CAD build for the part. Positions are in the model's coordinates, mm. Coordinates: 2 decimals unless noted, no trailing zeros. Order: outer loops, then holes, each group sorted by start corner. A loop starts at its lowest first (then second) coordinate and runs counter-clockwise, first axis right, second up. Notation, with made-up numbers: M -9.5,40.25 L -3.5,40.25 A11 cw -3.5,53.25 Z; hole C -14,36.25 d10. An arc over 180 degrees is marked long. Write item = value, one per line. Start each with the question number.
```python
from build123d import *

# Parameters (mm, degrees)
SKETCH1_R           = 317.5
SKETCH1_R_2         = 47.5
BOSS_EXTRUDE1_DEPTH = 5
SKETCH2_R           = 6
CUT_EXTRUDE1_DEPTH  = 5
CIRPATTERN1_COUNT   = 12
SKETCH6_R           = 3
CUT_EXTRUDE2_DEPTH  = 10
CIRPATTERN2_COUNT   = 3


with BuildPart() as part:
    # Sketch1 → Boss-Extrude1 (new body)
    with BuildSketch(Plane(origin=(0, 0, 0), x_dir=(0, 0, -1), z_dir=(1, 0, 0))):
        Circle(SKETCH1_R)
        Circle(SKETCH1_R_2, mode=Mode.SUBTRACT)
    extrude(amount=BOSS_EXTRUDE1_DEPTH)

    # Sketch2 → Cut-Extrude1 (cut)
    with BuildSketch(Plane(origin=(5, 0, 0), x_dir=(0, 0, -1), z_dir=(1, 0, 0))):
        with Locations((300, 0)):
            Circle(SKETCH2_R)
    cut_extrude1 = extrude(amount=-CUT_EXTRUDE1_DEPTH, mode=Mode.SUBTRACT)

    # CirPattern1: Cut-Extrude1 ×12 about axis
    cirpattern1_axis = Axis((0, 0, 0), (1, 0, 0))
    for i in range(1, CIRPATTERN1_COUNT):
        add(cut_extrude1.rotate(cirpattern1_axis, i * 360 / CIRPATTERN1_COUNT), mode=Mode.SUBTRACT)

    # Sketch6 → Cut-Extrude2 (cut)
    with BuildSketch(Plane(origin=(5, 0, 0), x_dir=(0, 0, -1), z_dir=(1, 0, 0))):
        with Locations((0, 55)):
            Circle(SKETCH6_R)
    cut_extrude2 = extrude(amount=-CUT_EXTRUDE2_DEPTH, mode=Mode.SUBTRACT)

    # CirPattern2: Cut-Extrude2 ×3 about axis
    cirpattern2_axis = Axis((0, 0, 0), (1, 0, 0))
    for i in range(1, CIRPATTERN2_COUNT):
        add(cut_extrude2.rotate(cirpattern2_axis, i * 360 / CIRPATTERN2_COUNT), mode=Mode.SUBTRACT)


solid = part.part
```
1. Probe L1, parallel to Y at x = 3, z = 5.5; L2, parallel to Y at x = 2.9, z = 150; L3, parallel to Y at x = 2.1, z = 43. List the from-to ranges inside material, lowest first.
2. Flat gauge pins, fed straight in: pin 1 (7 mm diameter, centred on y = -27.5, z = -47.63, fed in from -X); pin 2 (1.5 mm diameter, centred on x = 4, y = 171.5, fed in from -Z); pin 3 (1 mm diameter, centred on x = 1, z = 212.5, fed in from +Y); pin 4 (1 mm diameter, centred on x = 1.5, y = -27, fed in from +Z). Where does each tip first touch, or does it go through?
3. Slice it at A-A (x = 0.9). Give the number of separate pieces and of enclosed holes in the cut face, plus the area to 3 significant figures.
4. Slice it at C-C (y = -188.5). Write the cut outline in (x, z), plus the area to 3 significant figures.
5. Slice it at B-B (z = -242). Write the cut outline in (x, y).
Calculated:
q1.L1 = -317.45 to -302.4, -297.6 to -47.18, 47.18 to 297.6, 302.4 to 317.45
q1.L2 = -279.83 to -265.81, -253.81 to 253.81, 265.81 to 279.83
q1.L3 = -314.57 to -20.18, 20.18 to 314.57
q2.pin_1 = 0
q2.pin_2 = -267.68
q2.pin_3 = 236.35
q2.pin_4 = 316.39
q3.separate_pieces = 1
q3.enclosed_holes = 16
q3.area = 308,000 mm²
q4.outline = M 0,-255.49 L 5,-255.49 L 5,255.49 L 0,255.49 Z
q4.area = 2,550 mm²
q5.outline = M 0,-205.53 L 5,-205.53 L 5,205.53 L 0,205.53 Z
